Work out the finished part from the listing and answer in its coordinate system (mm). Face numbers are marked on the shaded views. Coordinates: 2 decimals unless noted, no trailing zeros. Order: outer loops, then holes, each group sorted by start corner. A loop starts at its lowest first (then second) coordinate and runs counter-clockwise, first axis right, second up. Notation, with made-up numbers: M 12,79 L 49,79 A25 cw 49,96 Z; hole C 86,25 d2. An arc over 180 degrees is marked long. Answer in a Markdown table with one row per item. Add a question column.
Item 1: The part is cut by section A-A (y = 21.59). Write down the section's boundary in (x, z).
Item 2: The part is cut by section B-B (z = 18.5). Write down the section's boundary in (x, y) (3 decimals), then the cut area to 3 significant figures.
Item 3: The mould has two halves that part along Y. Classify the marked faces 1, 2, 3 and 4: released by +Y, released by -Y, zero draft, split by the parting line, or undercut.
Item 4: The part is cut by section C-C (x = -31). State how many separate pieces and enclosed holes the cut face has, then the cut area to 3 significant figures.
Item 5: A flat-ended cylindrical pin translates along its axis: pin 1 Ø6.5 at (x, y) = (-32.24, 8.89) entering from +Z. Find the tip coordinate at first contact, or state that the pin passes through.
Item 6: Consider line 1 (Y direction, x = -32, z = 12.5) (3 decimals); line 2 (Y direction, x = -33, z = -17.5) (3 decimals); line 3 (X direction, y = 9.25, z = -6). Determine where each line is inside the solid, lowest interval first. Write a range as from..to.
from build123d import *

# Parameters (mm, degrees)
SKETCH1_W           = 19.05
SKETCH1_H           = 44.45
BOSS_EXTRUDE1_DEPTH = 28.575
SKETCH3_R           = 2.794
CUT_EXTRUDE2_DEPTH  = 68.236705218
CHAMFER2_SIZE       = 1.27


with BuildPart() as part:
    # Sketch1 → Boss-Extrude1 (new body)
    with BuildSketch(Plane(origin=(0, 0, 0), x_dir=(1, 0, 0), z_dir=(0, 1, 0))):
        with Locations((-32.049528302, -0.918054245)):
            Rectangle(SKETCH1_W, SKETCH1_H)
    extrude(amount=BOSS_EXTRUDE1_DEPTH)

    # Sketch3 → Cut-Extrude2 (cut, through all)
    with BuildSketch(Plane.XY.offset(23.143054245)):
        with Locations((-32.240028302, 34.29)):
            Circle(SKETCH3_R)
        with Locations((-32.240028302, 21.59)):
            Circle(SKETCH3_R)
        with Locations((-32.240028302, 8.89)):
            Circle(SKETCH3_R)
    extrude(amount=-CUT_EXTRUDE2_DEPTH, mode=Mode.SUBTRACT)

    # Chamfer2
    chamfer2_edges = [part.edges().sort_by_distance(p)[0] for p in [
        (-32.049528302, 28.575, 23.143054245),
        (-22.524528302, 28.575, 0.918054245),
        (-35.034028302, 21.59, -21.306945755),
        (-35.034028302, 21.59, 23.143054245),
        (-35.034028302, 8.89, -21.306945755),
        (-35.034028302, 8.89, 23.143054245),
        (-32.049528302, 28.575, -21.306945755),
        (-22.524528302, 14.2875, -21.306945755),
        (-22.524528302, 14.2875, 23.143054245),
        (-41.574528302, 14.2875, 23.143054245),
        (-41.574528302, 14.2875, -21.306945755),
        (-41.574528302, 28.575, 0.918054245),
    ]]
    chamfer(chamfer2_edges, length=CHAMFER2_SIZE)


solid = part.part
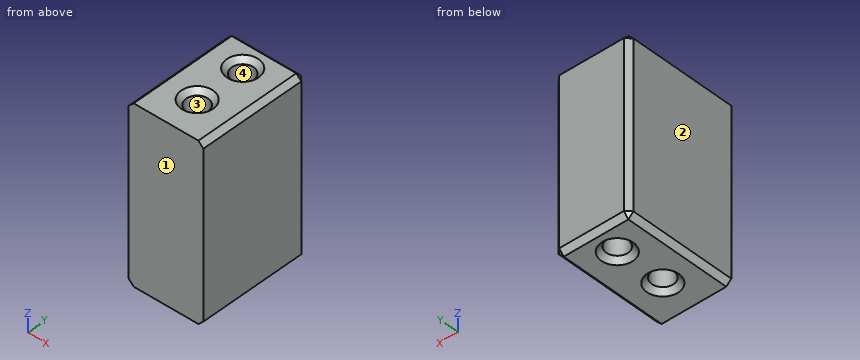
Reply:
| question | item | result |
|---|---|---|
| 1 | outline | M -41.57,-20.04 L -40.3,-21.31 L -36.3,-21.31 L -35.03,-20.04 L -35.03,21.87 L -36.3,23.14 L -40.3,23.14 L -41.57,21.87 Z; M -29.45,-20.04 L -28.18,-21.31 L -23.79,-21.31 L -22.52,-20.04 L -22.52,21.87 L -23.79,23.14 L -28.18,23.14 L -29.45,21.87 Z |
| 2 | outline | M -41.575,0 L -22.525,0 L -22.525,27.305 L -23.795,28.575 L -40.305,28.575 L -41.575,27.305 Z; hole C -32.24,8.89 d5.588; hole C -32.24,21.59 d5.588 |
| 2 | area | 494 mm2 |
| 3 | face 1 | released by -Y |
| 3 | face 2 | zero draft |
| 3 | face 3 | undercut |
| 3 | face 4 | undercut |
| 4 | separate pieces | 3 |
| 4 | enclosed holes | 0 |
| 4 | area | 816 mm2 |
| 5 | pin 1 | stops at z = 22.33 |
| 6 | line 1 | y = 0..6.106, 11.674..18.806, 24.374..28.575 |
| 6 | line 2 | y = 0..6.201, 11.579..18.901, 24.279..28.575 |
| 6 | line 3 | x = -41.57..-35.01, -29.47..-22.52 |
